from build123d import *

# Parameters (mm, degrees)
BOSS_EXTRUDE1_DEPTH      = 2
BOSS_EXTRUDE1_DEPTH_BACK = 4
BOSS_EXTRUDE2_DEPTH      = 2
BOSS_EXTRUDE3_DEPTH      = 2


with BuildPart() as part:
    # Sketch1 → Boss-Extrude1 (new body, two sides)
    with BuildSketch(Plane(origin=(0, 0, 0), x_dir=(0, 0, -1), z_dir=(1, 0, 0))) as boss_extrude1_sk:
        with BuildLine():
            Line((-6.25, 0), (-4.25, 0))
            ThreePointArc((-4.25, 0), (0, 4.25), (4.25, 0))
            ThreePointArc((4.25, 0), (4.213640661, -0.554736317), (4.105184762, -1.099980942))
            Line((4.105184762, -1.099980942), (6.037036414, -1.617619032))
            ThreePointArc((6.037036414, -1.617619032), (6.196530384, -0.815788701), (6.25, 0))
            ThreePointArc((6.25, 0), (0, 6.25), (-6.25, 0))
        make_face()
        with BuildLine():
            Line((6.037036414, -1.617619032), (4.105184762, -1.099980942))
            ThreePointArc((4.105184762, -1.099980942), (4.812291543, -2.324725813), (6.037036414, -1.617619032))
        make_face()
        with BuildLine():
            ThreePointArc((-4.105184762, -1.099980942), (-4.213640661, -0.554736317), (-4.25, 0))
            Line((-4.25, 0), (-6.25, 0))
            ThreePointArc((-6.25, 0), (-6.196530384, -0.815788701), (-6.037036414, -1.617619032))
            Line((-6.037036414, -1.617619032), (-5.071110588, -1.358799987))
            Line((-5.071110588, -1.358799987), (-4.105184762, -1.099980942))
        make_face()
        with BuildLine():
            ThreePointArc((-6.037036414, -1.617619032), (-4.812291543, -2.324725813), (-4.105184762, -1.099980942))
            Line((-4.105184762, -1.099980942), (-5.071110588, -1.358799987))
            Line((-5.071110588, -1.358799987), (-6.037036414, -1.617619032))
        make_face()
    extrude(amount=BOSS_EXTRUDE1_DEPTH)
    extrude(boss_extrude1_sk.sketch, amount=-BOSS_EXTRUDE1_DEPTH_BACK)

    # Sketch2 → Boss-Extrude2 (add)
    with BuildSketch(Plane(origin=(0, 0, 0), x_dir=(0, 0, -1), z_dir=(1, 0, 0))):
        Polygon((-2, 4.25), (0, 4.25), (2, 4.25), (2, 56.25), (-2, 56.25), align=None)
    extrude(amount=BOSS_EXTRUDE2_DEPTH)

    # Sketch3 → Boss-Extrude3 (add)
    with BuildSketch(Plane(origin=(0, 0, 0), x_dir=(0, 0, -1), z_dir=(1, 0, 0))):
        Polygon((1, 56.25), (0, 56.25), (-1, 56.25), (-1, 4.25), (1, 4.25), align=None)
    extrude(amount=-BOSS_EXTRUDE3_DEPTH)


solid = part.part
Source: CAD feature listing. Evaluate the final solid. Frame: model axes, mm. A direction names the side the tool comes from. Give positions to 0.01 mm unless a question says otherwise; leave off trailing zeros. Write each loop counter-clockwise with the first axis right and the second up, starting at its lowest first coordinate (ties: lowest second). Pieces come first, ordered by that corner, then holes. Notation, with made-up numbers: M 64.5,6 L 70.5,6 A9 ccw 70.5,20 Z; hole C -15.75,8 d7. An arc over 180 degrees is marked long. Answer as a JSON object with one key per item and string values.
Q1. Contact query for flat-ended pins moving along their axis: P1, Ø0.6, axis at x = 1.5, y = 28.5, coming from the -Z side; P2, Ø0.6, axis at x = 1, y = 35, coming from the +Z side; P3, Ø1.1, axis at y = 41, z = 1.5, coming from the -X side; P4, Ø2, axis at y = 22.5, z = 3.5, coming from the -X side. Output: stop coordinate, or through.
Geometry check:
{"P1": "stops at z = -2", "P2": "stops at z = 2", "P3": "stops at x = -2", "P4": "passes through"}
Q2. Cut plane A-A, the plane y = 10.5. Return the cut outline in (x, z).
Geometry check:
{"outline": "M -2,-1 L 0,-1 L 0,-2 L 2,-2 L 2,2 L 0,2 L 0,1 L -2,1 Z"}
Q3. Mould query, pull axis Z, two halves, no side actions, for faces 1 (the face through (-1, 32, 1)), 2 (the face through (-1, 31, -1)), 3 (the face through (-4, 5, 0)), 4 (the face through (-1.04, -2.32, -4.79)). Classes: +Z half, -Z half, draft (parallel to the pull), parting line (faces both ways), or undercut.
Geometry check:
{"face 1": "+Z half", "face 2": "-Z half", "face 3": "draft", "face 4": "undercut"}
Q4. Cut plane C-C, the plane x = -1. Return the cut outline in (y, z), then the cut area to 3 significant figures.
Geometry check:
{"outline": "M -1.62,-6.04 A6.25 ccw 6.17,-1 L 56.25,-1 L 56.25,1 L 6.17,1 A6.25 ccw -1.62,6.04 A1 ccw -1.1,4.11 A4.25 cw long -1.1,-4.11 A1 ccw Z", "area": "142 mm^2"}
Q5. Ray query, line 1 along Y through (x, z) = (-1.55, 0); line 2 along Z through (x, y) = (1.6, 18.5). Return the intervals inside material, ascending.
Geometry check:
{"line 1": "y = 4.25 to 56.25", "line 2": "z = -2 to 2"}
Q6. Access query for faces 5 (the face through (0, 31.4, -1.5)), 6 (the face through (0, 31.4, 1.5)), 7 (the face through (1, 31, -2)), 8 (the face through (1, 31, 2)). Directions: +Z, -Z, +X, -X, +Y, -Y. A direction counts if a zero-diameter tool reaches every point of the face in a straight line with its end or side. Return the directions, or none.
Geometry check:
{"face 5": "-Z, -X, +Y", "face 6": "+Z, -X, +Y", "face 7": "-Z, +X, -X, +Y", "face 8": "+Z, +X, -X, +Y"}
Q7. Cut plane B-B, the plane z = 0. Return the cut outline in (x, y).
Geometry check:
{"outline": "M -4,4.25 L 2,4.25 L 2,56.25 L -2,56.25 L -2,6.25 L -4,6.25 Z"}
Q8. Cut plane D-D, the plane x = -3.4. Return the cut outline in (y, z).
Geometry check:
{"outline": "M -1.62,-6.04 A6.25 ccw long -1.62,6.04 A1 ccw -1.1,4.11 A4.25 cw long -1.1,-4.11 A1 ccw Z"}
